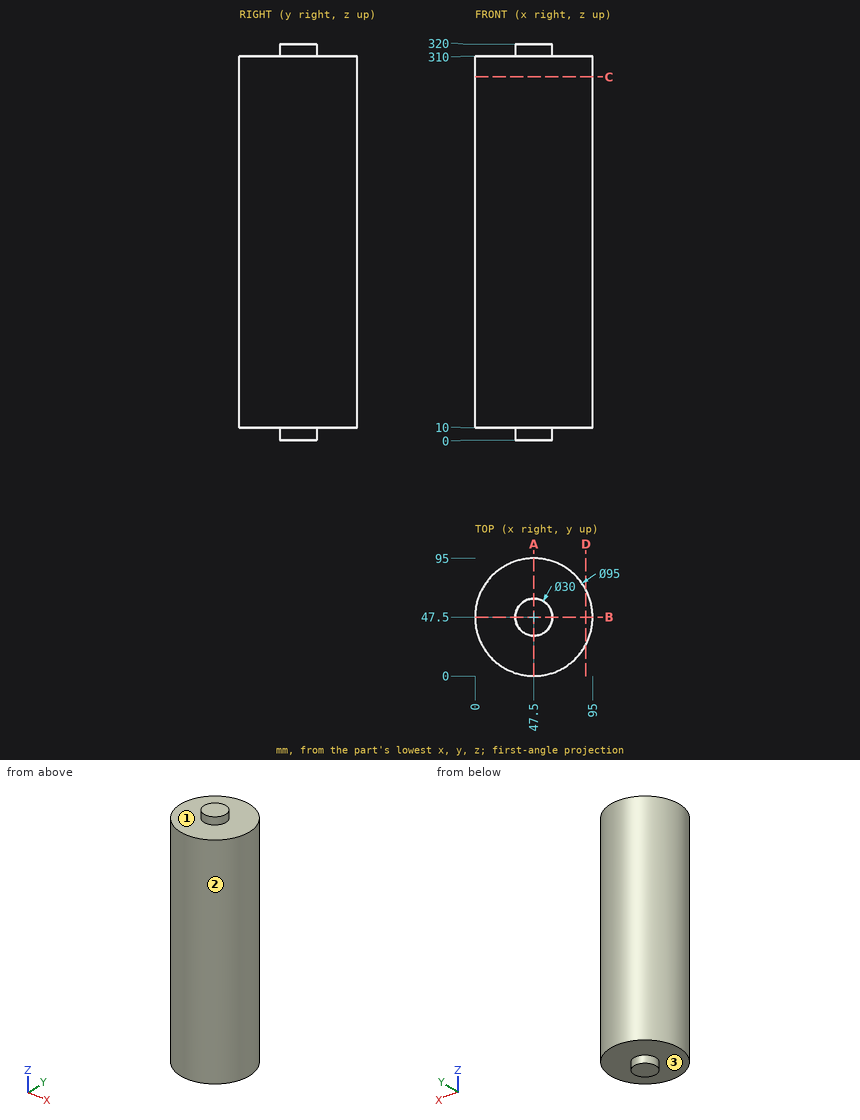
Could you check a few things on this drawing? It's one solid part, dimensions in mm from its lowest x, y, z. A direction names the side the tool comes from. Coordinates: 2 decimals unless noted, no trailing zeros. Order: outer loops, then holes, each group sorted by start corner. A loop starts at its lowest first (then second) coordinate and runs counter-clockwise, first axis right, second up.
1. If we section it at A-A (x = 47.5): Please give me the cut outline in (y, z).
2. If we section it at D-D (x = 89.5): Please give me the cut outline in (y, z), then the cut area to 3 significant figures.
3. If we section it at C-C (z = 293.5): Please give me the cut outline in (x, y), then the cut area to 3 significant figures.
4. I need wall thicknesses on line 1 (Z direction, x = 10, y = 38.5); line 2 (X direction, y = 47, z = 131); line 3 (X direction, y = 50, z = 264). Which ranges of each line are inside material? Lowest first, please.
5. For the marked faces 1, 2 and 3, which set-ups out of +Z, -Z, +X, -X, +Y, -Y let a thin tool reach every point of the face, with its end or its side?
6. I'm going to push flat-ended pins straight in: pin 1 (4 mm diameter, centred on x = 27.5, y = 57.5, fed in from -Z); pin 2 (5 mm diameter, centred on x = 82, z = 122, fed in from +Y); pin 3 (6 mm diameter, centred on x = 22.5, z = 171.5, fed in from -Y). Where does each tip first touch, or does it pass through?
Entries:
1. outline: (0, 10) - (32.5, 10) - (32.5, 0) - (62.5, 0) - (62.5, 10) - (95, 10) - (95, 310) - (62.5, 310) - (62.5, 320) - (32.5, 320) - (32.5, 310) - (0, 310) - close
2. outline: (25.31, 10) - (69.69, 10) - (69.69, 310) - (25.31, 310) - close
2. area: 13,300 mm2
3. outline: circle Ø95 at (47.5, 47.5)
3. area: 7,090 mm2
4. line 1: z = 10 to 310
4. line 2: x = 0 to 95
4. line 3: x = 0.07 to 94.93
5. face 1: +Z
5. face 2: +Z, -Z
5. face 3: -Z
6. pin 1: stops at z = 10
6. pin 2: stops at y = 82.6
6. pin 3: stops at y = 5.4
